The model under review builds one solid part; all positions refer to its coordinate system, in mm. Give positions to 0.01 mm unless a question says otherwise; leave off trailing zeros. Order: outer loops, then holes, each group sorted by start corner. A loop starts at its lowest first (then second) coordinate and runs counter-clockwise, first axis right, second up. Notation, with made-up numbers: (-18.5, 0) - (40.5, 0) arc R6 ccw to (40.5, 4) - close; hole circle Ø10 at (31.25, 87.25). An arc over 180 degrees is marked (long way). Put each result on its own line as item: value.
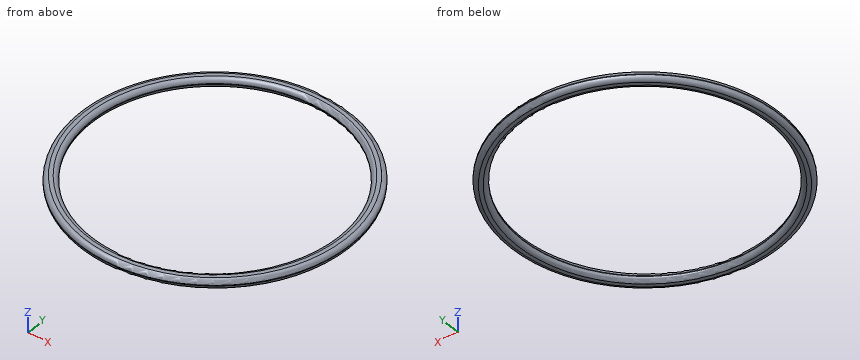
```python
from build123d import *

# Parameters (mm, degrees)
SKETCH017_R   = 11
SKETCH017_R_2 = 10
PAD007_DEPTH  = 0.75
FILLET006_R   = 0.35
FILLET007_R   = 0.35
FILLET008_R   = 0.35
FILLET009_R   = 0.35


with BuildPart() as part:
    # Sketch017 → Pad007 (new body)
    with BuildSketch(Plane.XY):
        Circle(SKETCH017_R)
        Circle(SKETCH017_R_2, mode=Mode.SUBTRACT)
    extrude(amount=PAD007_DEPTH)

    # Fillet006
    fillet006_edges = [part.edges().sort_by_distance(p)[0] for p in [
        (-11, 0, 0.75),
    ]]
    fillet(fillet006_edges, radius=FILLET006_R)

    # Fillet007
    fillet007_edges = [part.edges().sort_by_distance(p)[0] for p in [
        (-11, 0, 0),
    ]]
    fillet(fillet007_edges, radius=FILLET007_R)

    # Fillet008
    fillet008_edges = [part.edges().sort_by_distance(p)[0] for p in [
        (-10, 0, 0.75),
    ]]
    fillet(fillet008_edges, radius=FILLET008_R)

    # Fillet009
    fillet009_edges = [part.edges().sort_by_distance(p)[0] for p in [
        (-10, 0, 0),
    ]]
    fillet(fillet009_edges, radius=FILLET009_R)


with BuildPart() as part_1:
    # Body005 placement: moved
    add(part.part.moved(Location((0, 1e-05, 76.39999))))


solid = part_1.part
```
(1) Take a section at B-B, the plane z = 76.6. Write out the cut boundary in (x, y), then the cut area to 3 significant figures.
The answers:
outline: circle Ø21.93 at (0, 0); hole circle Ø20.07 at (0, 0)
area: 61.5 mm^2
(2) Wall thickness on L1, parallel to Y at x = 0, z = 76.8; L2, parallel to X at y = -1.5, z = 77.1; L3, parallel to Y at x = -2.5, z = 76.7: over which ranges is each line inside the solid? List them lowest first.
The answers:
L1: -11 to -10, 10 to 11
L2: -10.73 to -10.06, 10.06 to 10.73
L3: -10.71 to -9.69, 9.69 to 10.71
(3) Take a section at A-A, the plane x = 0. Write out the cut boundary in (y, z).
The answers:
outline: (-11, 76.75) arc R0.35 ccw to (-10.65, 76.4) - (-10.35, 76.4) arc R0.35 ccw to (-10, 76.75) - (-10, 76.8) arc R0.35 ccw to (-10.35, 77.15) - (-10.65, 77.15) arc R0.35 ccw to (-11, 76.8) - close; (10, 76.75) arc R0.35 ccw to (10.35, 76.4) - (10.65, 76.4) arc R0.35 ccw to (11, 76.75) - (11, 76.8) arc R0.35 ccw to (10.65, 77.15) - (10.35, 77.15) arc R0.35 ccw to (10, 76.8) - close
